Could you check a few things on this drawing? It's one solid part, dimensions in mm from its lowest x, y, z. Give positions to 0.01 mm unless a question says otherwise; leave off trailing zeros. Order: outer loops, then holes, each group sorted by start corner. A loop starts at its lowest first (then second) coordinate and runs counter-clockwise, first axis right, second up. Notation, with made-up numbers: (-17.75, -24) -> (-3.75, -24) arc R20 ccw to (-3.75, 0) -> close; hole circle Ø11 at (48, 6). An arc over 180 degrees is marked (long way). Answer as CSV lines item,"result".
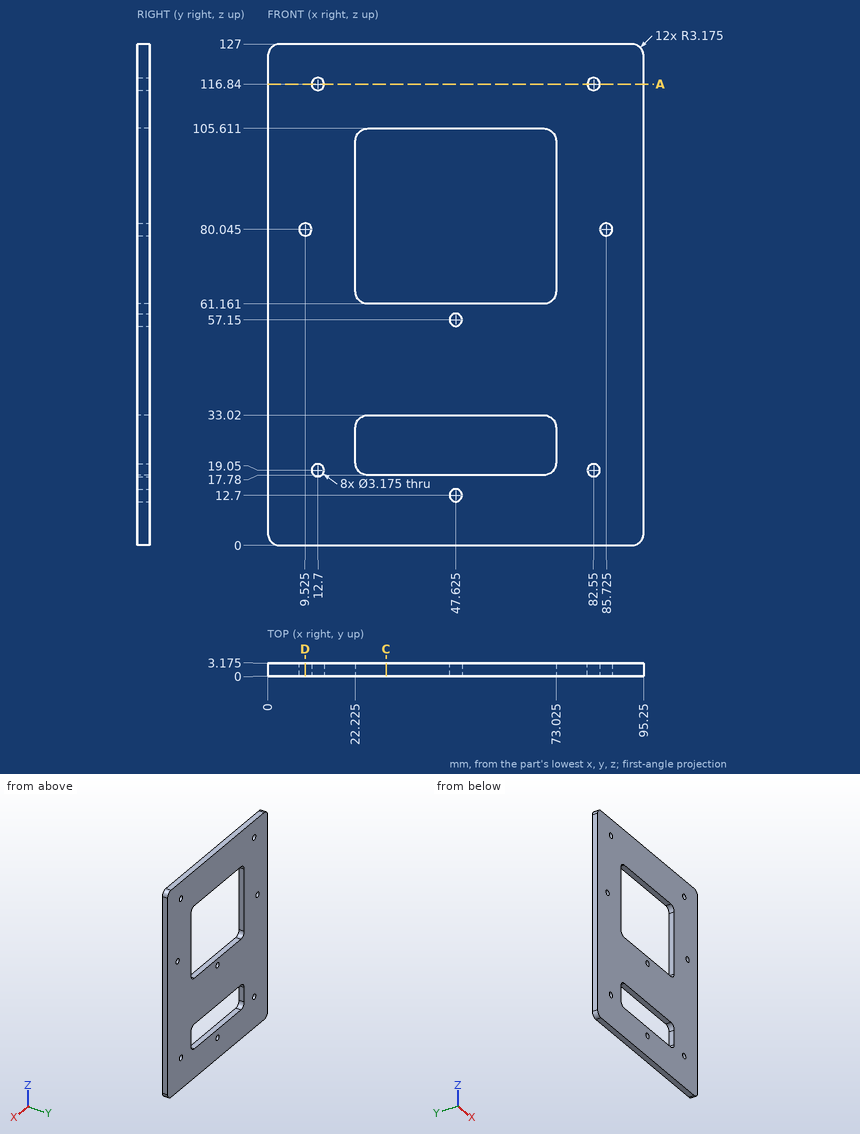
Item 1: Imagine slicing it at C-C, the plane x = 30. Please give me the cut outline in (y, z) (1 decimal).
Numbers:
outline,"(0, 0) -> (3.2, 0) -> (3.2, 17.8) -> (0, 17.8) -> close; (0, 33) -> (3.2, 33) -> (3.2, 61.2) -> (0, 61.2) -> close; (0, 105.6) -> (3.2, 105.6) -> (3.2, 127) -> (0, 127) -> close"
Item 2: Imagine slicing it at D-D, the plane x = 9.5. Please give me the cut outline in (y, z) (1 decimal), then the cut area to 3 significant figures.
Numbers:
outline,"(0, 0) -> (3.2, 0) -> (3.2, 78.5) -> (0, 78.5) -> close; (0, 81.6) -> (3.2, 81.6) -> (3.2, 127) -> (0, 127) -> close"
area,"393 mm²"
Item 3: Imagine slicing it at A-A, the plane z = 116.84. Give the number of separate pieces and of enclosed holes in the cut face, then the cut area to 3 significant figures.
Numbers:
separate pieces,"3"
enclosed holes,"0"
area,"282 mm²"
Item 4: Please list where these lines run through material, in increasing order: line 1 along Z through (x, y) = (32, 2.2); line 2 along Z through (x, y) = (12.7, 1.9); line 3 along X through (y, z) = (2.85, 117).
Numbers:
line 1,"z = 0 to 17.78, 33.02 to 61.16, 105.61 to 127"
line 2,"z = 0 to 17.46, 20.64 to 115.25, 118.43 to 127"
line 3,"x = 0 to 11.12, 14.28 to 80.97, 84.13 to 95.25"
